The model under review builds one solid part; all positions refer to its coordinate system, in mm. Coordinates: 2 decimals unless noted, no trailing zeros. Order: outer loops, then holes, each group sorted by start corner. A loop starts at its lowest first (then second) coordinate and runs counter-clockwise, first axis right, second up. Notation, with made-up numbers: M -16.75,6.5 L 37.25,6.5 A20 cw 37.25,27.5 Z; hole C 79,60 d7. An arc over 180 degrees is marked long. Answer as CSV lines item,"result". Start each with the question number.
Q1. Wall thickness on L1, parallel to Y at x = -7, z = 483 (3 decimals); L2, parallel to X at y = 31.5, z = 547 (3 decimals); L3, parallel to Y at x = -16, z = 386.5 (3 decimals): over which ranges is each line inside the solid? List them lowest first. Write a range as [from, to].
Q2. Consider section B-B on z = 470.5. Write out the cut boundary in (x, y) (3 decimals).
Q3. For P1, Ø17.5, axis at x = -14, z = 421.5, coming from the -Y side; P2, Ø8, axis at x = -9, y = 39, coming from the +Z side; P3, Ø12.5, axis at y = 38, z = 626.5, coming from the -X side (3 decimals), all flat-tipped, find the tip position at first contact; note any pin that passes through.
Q4. Consider section C-C on y = 35. Write out the cut boundary in (x, z) (3 decimals), and give its area (3 significant figures).
Q5. Consider section D-D on x = 15. Write out the cut boundary in (y, z), and give its area (3 significant figures).
Autodesk Inventor part; units mm, degrees
ref_plane "YZ Plane" through (0, 0, 0) normal (1, 0, 0) x (0, 1, 0)
ref_plane "XZ Plane" through (0, 0, 0) normal (0, 1, 0) x (-1, 0, 0)
ref_plane "XY Plane" through (0, 0, 0) normal (0, 0, 1) x (1, 0, 0)
sketch "Sketch1" plane through (0, 0, 0) normal (0, 0, 1) x (1, 0, 0)
  line L0 (19.05, -44.45) -> (-19.05, -44.45)
  line L1 (-19.05, -44.45) -> (-19.05, 44.45)
  line L2 (-19.05, 44.45) -> (19.05, 44.45)
  line L3 (19.05, 44.45) -> (19.05, -44.45)
  line L4 (19.05, -44.45) -> (-19.05, 44.45) construction
  line L5 (-19.05, -44.45) -> (19.05, 44.45) construction
  point P0 (0, 0)
  dimension "d0" = 38.1
  dimension "d1" = 88.9
extrude "Extrusion1" add sketch "Sketch1" along normal blind 673.8874
sketch "Sketch2" plane through (0, 0, 673.8874) normal (0, 0, 1) x (1, 0, 0)
  line L0 (19.05, -44.45) -> (19.05, 44.45)
  line L1 (19.05, 44.45) -> (-19.05, 44.45)
  line L2 (19.05, 31.75) -> (3.175, 31.75)
  line L3 (3.175, 31.75) -> (3.175, 28.575)
  line L4 (3.175, 28.575) -> (19.05, 28.575)
  line L5 (19.05, 28.575) -> (19.05, 31.75)
  line L6 (-19.05, 44.45) -> (-19.05, -44.45)
  line L7 (0, 25.0075) -> (0, 34.7359)
  line L8 (-19.05, 31.75) -> (-3.175, 31.75)
  line L9 (-3.175, 31.75) -> (-3.175, 28.575)
  line L10 (-3.175, 28.575) -> (-19.05, 28.575)
  line L11 (-19.05, 28.575) -> (-19.05, 31.75)
  point P0 (0, 0)
  dimension "d4" = 12.7
  dimension "d5" = 3.175
  dimension "d6" = 15.875
sketch "Sketch4" plane through (19.05, -44.45, 673.8874) normal (1, 0, 0) x (0, 0, -1)
  line L0 (0, 0) -> (0, 88.9)
  line L1 (673.8874, 0) -> (0, 0)
  line L2 (673.8874, 88.9) -> (673.8874, 0)
  line L3 (673.8874, 6.35) -> (0, 6.35)
  line L4 (152.4, 6.35) -> (0, 47.1855)
  line L5 (250.444, 6.35) -> (421.8705, 26.67)
  line L6 (421.8705, 26.67) -> (673.8874, 26.67)
  point P0 (673.8874, 73.025)
  point P1 (0, 73.025)
  point P2 (673.8874, 44.45)
  dimension "d15" = 6.35
  dimension "d20" = 152.4
  dimension "d21" = 165
  dimension "d23" = 20.32
  dimension "d24" = 98.044
  dimension "d25" = 173.24
extrude "Extrusion3" cut sketch "Sketch4" against normal blind 152.4
sketch "Sketch5" plane through (-19.05, 44.45, 0) normal (0, 1, 0) x (1, 0, 0)
  line L0 (38.1, -673.8874) -> (15.875, -673.8874)
  line L1 (15.875, -673.8874) -> (15.875, -572.2874)
  line L2 (15.875, -572.2874) -> (38.1, -572.2874)
  line L3 (38.1, -572.2874) -> (38.1, -673.8874)
  line L4 (19.05, -558.0239) -> (19.05, -615.4069)
  line L5 (0, -673.8874) -> (22.225, -673.8874)
  line L6 (22.225, -673.8874) -> (22.225, -572.2874)
  line L7 (22.225, -572.2874) -> (0, -572.2874)
  line L8 (0, -572.2874) -> (0, -673.8874)
  point P0 (19.05, 0)
  dimension "d28" = 22.225
  dimension "d29" = 101.6
extrude "Extrusion4" cut sketch "Sketch5" against normal blind 15.875 contours L0 L1 L2 L6 | L5 L8 L7 L1
sketch "Sketch6" plane through (-19.05, 44.45, 0) normal (0, 1, 0) x (1, 0, 0)
  line L0 (38.1, 0) -> (38.1, -673.8874)
  line L1 (0, 0) -> (38.1, 0)
  line L2 (38.1, -215.9) -> (0, -215.9)
  line L3 (0, -215.9) -> (0, -342.9)
  line L4 (0, -342.9) -> (38.1, -342.9)
  line L5 (38.1, -342.9) -> (38.1, -215.9)
  point P0 (38.1, -572.2874)
  point P1 (19.05, 0)
  dimension "d32" = 127
  dimension "d33" = 215.9
  dimension "d36" = 38.1
extrude "Extrusion5" cut sketch "Sketch6" against normal blind 15.875
sketch "Sketch7" plane through (0, 0, 0) normal (0, 0, -1) x (-1, 0, 0)
  line L0 (41.2519, 59.9443) -> (-67.5031, 59.9443)
  line L1 (-67.5031, 59.9443) -> (-67.5031, -55.7754)
  line L2 (-67.5031, -55.7754) -> (41.2519, -55.7754)
  line L3 (41.2519, -55.7754) -> (41.2519, 59.9443)
  point P0 (0, 0)
extrude "Extrusion6" cut sketch "Sketch7" against normal blind 342.9
extrude "Extrusion7" cut sketch "Sketch2" against normal blind 508 contours L8 L9 L10 L6
properties part number "FrontSkidRight"
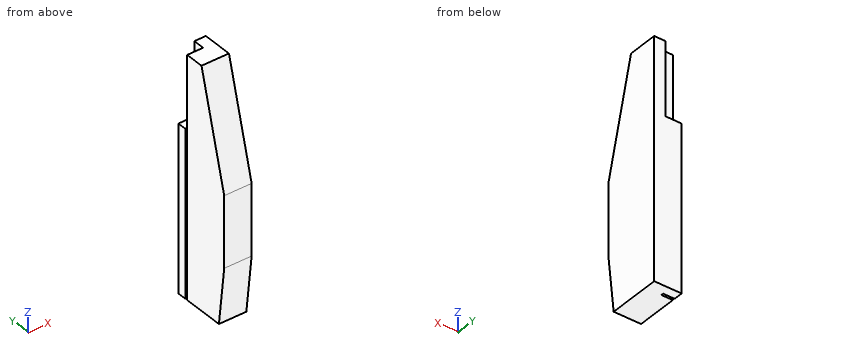
Evaluation:
1,L1,"y = [-38.1, 28.575], [31.75, 44.45]"
1,L2,"x = [-3.175, 19.05]"
1,L3,"y = [-33.721, 28.575], [31.75, 44.45]"
2,outline,"M -19.05,-38.1 L 19.05,-38.1 L 19.05,44.45 L -19.05,44.45 L -19.05,31.75 L -3.175,31.75 L -3.175,28.575 L -19.05,28.575 Z"
3,P1,"stops at y = -38.1"
3,P2,"stops at z = 572.29"
3,P3,"stops at x = 3.175"
4,outline,"M -19.05,342.9 L 19.05,342.9 L 19.05,673.887 L 3.175,673.887 L 3.175,572.287 L -19.05,572.287 Z"
4,area,"10,400 mm²"
5,outline,"M -38.1,423.44 L -28.55,342.9 L 44.45,342.9 L 44.45,673.89 L 2.74,673.89 L -38.1,521.49 Z"
5,area,"23,800 mm²"
